Can you work these out from the model? Positions are in its coordinate system, mm. A direction names the side the tool comes from. Coordinates: 2 decimals unless noted, no trailing zeros. Order: outer loops, then holes, each group sorted by start corner. A loop starts at its lowest first (then second) coordinate and runs counter-clockwise, first axis right, second up. Notation, with made-up numbers: (59, 78) -> (90, 78) arc R16 ccw to (90, 93) -> close; hole circle Ø3 at (77.25, 8). An arc over 180 degrees is marked (long way). Answer in a Markdown table with one row per item.
```python
from build123d import *

# Parameters (mm, degrees)
SKETCH1_R               = 1.4
BOSS_EXTRUDE1_DEPTH     = 7
BOSS_EXTRUDE1_2_DEPTH   = 7
BOSS_EXTRUDE1_3_DEPTH   = 7
BOSS_EXTRUDE1_4_DEPTH   = 7
BOSS_EXTRUDE2_DEPTH     = 2.5
FILLET1_R               = 1
CUT_EXTRUDE1_DEPTH      = 28.434011737
CUT_EXTRUDE1_DEPTH_BACK = 28.434011737
SKETCH4_R               = 1
SKETCH5_R               = 2
CUT_EXTRUDE2_DEPTH      = 0.5


with BuildPart() as part:
    # Sketch1 → Boss-Extrude1 (new body)
    with BuildSketch(Plane(origin=(0, 0, 0), x_dir=(1, 0, 0), z_dir=(0, 1, 0))):
        with Locations(Location((-15.25, -15.25, 0), (0, 0, 270))):
            Circle(SKETCH1_R)
    extrude(amount=BOSS_EXTRUDE1_DEPTH)



with BuildPart() as body_2:
    # Sketch1 → Boss-Extrude1 2 (new body)
    with BuildSketch(Plane(origin=(0, 0, 0), x_dir=(1, 0, 0), z_dir=(0, 1, 0))):
        with Locations(Location((-15.25, 15.25, 0), (0, 0, 270))):
            Circle(SKETCH1_R)
    extrude(amount=BOSS_EXTRUDE1_2_DEPTH)


with BuildPart() as body_3:
    # Sketch1 → Boss-Extrude1 3 (new body)
    with BuildSketch(Plane(origin=(0, 0, 0), x_dir=(1, 0, 0), z_dir=(0, 1, 0))):
        with Locations(Location((15.25, 15.25, 0), (0, 0, 270))):
            Circle(SKETCH1_R)
    extrude(amount=BOSS_EXTRUDE1_3_DEPTH)


with BuildPart() as body_4:
    # Sketch1 → Boss-Extrude1 4 (new body)
    with BuildSketch(Plane(origin=(0, 0, 0), x_dir=(1, 0, 0), z_dir=(0, 1, 0))):
        with Locations(Location((15.25, -15.25, 0), (0, 0, 270))):
            Circle(SKETCH1_R)
    extrude(amount=BOSS_EXTRUDE1_4_DEPTH)


with BuildPart() as part_1:
    add(part.part)

    add(body_2.part)  # Boss-Extrude2 merges body 2

    add(body_3.part)  # Boss-Extrude2 merges body 3

    add(body_4.part)  # Boss-Extrude2 merges body 4
    # Sketch2 → Boss-Extrude2 (add)
    with BuildSketch(Plane.XZ):
        Polygon((-12.25, 12.25), (12.25, 12.25), (12.25, -18.25), (18.25, -18.25), (18.25, 19.25), (-18.25, 19.25), (-18.25, -18.25), (-12.25, -18.25), align=None)
    extrude(amount=BOSS_EXTRUDE2_DEPTH)

    # Fillet1
    fillet1_edges = [part_1.edges().sort_by_distance(p)[0] for p in [
        (-12.25, -2.5, -3),
        (0, -2.5, 12.25),
        (12.25, -2.5, -3),
        (15.25, -2.5, -18.25),
        (18.25, 0, 0.5),
        (18.25, -1.25, -18.25),
        (-18.25, 0, 0.5),
        (-15.25, 0, -18.25),
        (-18.25, -1.25, -18.25),
        (-12.25, 0, -3),
        (-12.25, -1.25, -18.25),
        (0, 0, 12.25),
        (12.25, 0, -3),
        (15.25, 0, -18.25),
        (12.25, -1.25, -18.25),
        (18.25, -2.5, 0.5),
        (-18.25, -2.5, 0.5),
        (-15.25, -2.5, -18.25),
    ]]
    fillet(fillet1_edges, radius=FILLET1_R)

    # Sketch4 → Cut-Extrude1 (cut, two sides: drawn at the far end of the back side and taken through both)
    with BuildSketch(Plane(origin=(0, 0, 0), x_dir=(1, 0, 0), z_dir=(0, 1, 0)).offset(-CUT_EXTRUDE1_DEPTH_BACK)):
        with Locations(Location((-12, -16.566325801, 0), (0, 0, 270))):
            Circle(SKETCH4_R)
        with Locations(Location((12, -16.566325801, 0), (0, 0, 270))):
            Circle(SKETCH4_R)
    extrude(amount=CUT_EXTRUDE1_DEPTH + CUT_EXTRUDE1_DEPTH_BACK, mode=Mode.SUBTRACT)

    # Sketch5 → Cut-Extrude2 (cut)
    with BuildSketch(Plane(origin=(0, 0, 0), x_dir=(1, 0, 0), z_dir=(0, 1, 0))):
        with Locations(Location((-12, -16.566325801, 0), (0, 0, 270))):
            Circle(SKETCH5_R)
        with Locations(Location((12, -16.566325801, 0), (0, 0, 270))):
            Circle(SKETCH5_R)
    extrude(amount=-CUT_EXTRUDE2_DEPTH, mode=Mode.SUBTRACT)


solid = part_1.part
```
(1) Suppose I cut it at A-A (z = -15.25). Please give me the cut outline in (x, y), and give its area (3 significant figures).
Response values:
| item | result |
|---|---|
| outline | (-18.25, -1.5) arc R1 ccw to (-17.25, -2.5) -> (-13.25, -2.5) arc R1 ccw to (-12.25, -1.5) -> (-12.25, -1) arc R1 ccw to (-13.25, 0) -> (-13.85, 0) -> (-13.85, 7) -> (-16.65, 7) -> (-16.65, 0) -> (-17.25, 0) arc R1 ccw to (-18.25, -1) -> close; (12.25, -1.5) arc R1 ccw to (13.25, -2.5) -> (17.25, -2.5) arc R1 ccw to (18.25, -1.5) -> (18.25, -1) arc R1 ccw to (17.25, 0) -> (16.65, 0) -> (16.65, 7) -> (13.85, 7) -> (13.85, 0) -> (13.25, 0) arc R1 ccw to (12.25, -1) -> close |
| area | 67.5 mm2 |
(2) Suppose I cut it at D-D (z = 11). Please give me the cut outline in (x, y).
Response values:
| item | result |
|---|---|
| outline | (-18.25, -1.5) arc R1 ccw to (-17.25, -2.5) -> (-13.25, -2.5) arc R1 ccw to (-12.25, -1.5) -> (-12.25, -1) arc R1 ccw to (-13.25, 0) -> (-17.25, 0) arc R1 ccw to (-18.25, -1) -> close; (12.25, -1.5) arc R1 ccw to (13.25, -2.5) -> (17.25, -2.5) arc R1 ccw to (18.25, -1.5) -> (18.25, -1) arc R1 ccw to (17.25, 0) -> (13.25, 0) arc R1 ccw to (12.25, -1) -> close |
(3) Suppose I cut it at B-B (y = 2). Please give me the cut outline in (x, z), and give its area (3 significant figures).
Response values:
| item | result |
|---|---|
| outline | circle Ø2.8 at (-15.25, -15.25); circle Ø2.8 at (-15.25, 15.25); circle Ø2.8 at (15.25, -15.25); circle Ø2.8 at (15.25, 15.25) |
| area | 24.6 mm2 |
(4) Will these pins go through, and if not, where does the flat tip stop? pin 1 Ø3 at (x, z) = (12, 17.5) entering from +Y; pin 2 Ø0.6 at (x, y) = (4, -1) entering from -Z; pin 3 Ø1.5 at (x, y) = (14.5, 3.5) entering from -Z.
Response values:
| item | result |
|---|---|
| pin 1 | y = 0 |
| pin 2 | z = 12.25 |
| pin 3 | z = -16.65 |
(5) On a 3-axis mill with a long thin cutter (end or side, diameter ignored), from which of +Z, -Z, +X, -X, +Y, -Y can I reach the whole of each face in a straight line? I mean faces 1 (the cylindrical face through (-12.535, -0.301, -1.787)), 2 (the cylindrical face through (-15.222, -0.285, -17.949)), 3 (the cylindrical face through (16.2, 3.45, -16.28)), 4 (the cylindrical face through (12.535, -2.199, -2.214)). Say none if no direction works.
Response values:
| item | result |
|---|---|
| face 1 | -Z, +Y |
| face 2 | -Z, +X, -X, +Y |
| face 3 | +Y |
| face 4 | -Z, -Y |
(6) Suppose I cut it at C-C (x = 8.5). Please give me the cut outline in (y, z), and give its area (3 significant figures).
Response values:
| item | result |
|---|---|
| outline | (-2.5, 13.25) arc R1 ccw to (-1.5, 12.25) -> (-1, 12.25) arc R1 ccw to (0, 13.25) -> (0, 19.25) -> (-2.5, 19.25) -> close |
| area | 17.1 mm2 |
(7) We'd pull the mould along X, two halves only. Please class faces 5 (the cylindrical face through (17.949, -2.215, 1.256)), 6 (the cylindrical face through (12.535, -0.301, -2.214)), 7 (the flat face through (0, -1, 19.25)): +X half, -X half, draft (parallel to the pull), parting line (faces both ways), or undercut.
Response values:
| item | result |
|---|---|
| face 5 | +X half |
| face 6 | undercut |
| face 7 | draft |
(8) I need wall thicknesses on line 1 (Z direction, x = -12, y = -1.65); line 2 (Z direction, x = -12, y = -1.5); line 3 (Y direction, x = -6.5, z = 15). Which ranges of each line are inside material? Lowest first, please. Write a range as [from, to].
Response values:
| item | result |
|---|---|
| line 1 | [12.26, 15.57], [17.57, 19.25] |
| line 2 | [12.25, 15.57], [17.57, 19.25] |
| line 3 | [-2.5, 0] |
